The model under review builds one solid part; all positions refer to its coordinate system, in mm. A direction names the side the tool comes from. Give positions to 0.01 mm unless a question says otherwise; leave off trailing zeros. Loops run counter-clockwise (first coordinate to the right, second up) from the corner with the lowest first, then second, coordinate; pieces in that order, holes last. Notation, with made-up numbers: M 22.5,28 L 28.5,28 A16 ccw 28.5,47 Z; hole C 28,-17 d10. An arc over 180 degrees is marked long. Write item = value, one per line. Start each with the question number.
1. We need section B-B on x = 7.5. Give the boundary of the cut face in (y, z).
2. Draft analysis for pull direction X (two halves, no side actions). For faces 6 (the face through (0, 1.5, 0)), 7 (the face through (0.1, 7.6, 0)), 8 (the face through (8.7, 2.34, -0.05)), 9 (the face through (-6.3, 2.34, -0.05)), state which applies: pulls with the +X half, pulls with the -X half, needs draft (parallel to the pull), parting line crosses it, or undercut.
3. Wall thickness on line 1 along Z through (x, y) = (-7.5, 2.45); line 2 along X through (y, z) = (4.5, -0.75); line 3 along X through (y, z) = (1, -0.75): over which ranges is each line inside the solid? List them lowest first. Write a range as from..to.
4. We need section C-C on z = -2.25. Give the boundary of the cut face in (x, y).
5. We need section A-A on x = -9. Give the boundary of the cut face in (y, z), then the cut area to 3 significant figures.
6. We need section D-D on y = 4.25. Give the boundary of the cut face in (x, z), then the cut area to 3 significant figures.
7. For faces 1 (the face through (6, 3.1, 0)), 2 (the face through (-2, 1, -3)), 3 (the face through (0, 6.1, 0)), 4 (the face through (0, 0, 0)), 5 (the face through (-9, 3.1, 0)), list the 3-axis set-ups (+Z, -Z, +X, -X, +Y, -Y) from which the entire face can be reached by the end or side of a thin tool; tool diameter is ignored.
8. For pin 1 (1.8 mm diameter, centred on x = 7, z = 0, fed in from +Y); pin 2 (1 mm diameter, centred on y = 5, z = -0.5, fed in from +X), all flat-tipped, find the tip position at first contact; note any pin that passes through.
from build123d import *

# Parameters (mm, degrees)
BOSS_EXTRUDE1_DEPTH  = 3
M2_CLEARANCE_HOLE1_D = 2.4
FILLET1_R            = 2


with BuildPart() as part:
    # Sketch1 → Boss-Extrude1 (new, symmetric)
    with BuildSketch(Plane.XY):
        with BuildLine():
            ThreePointArc((4.5, 3.1), (3.439339828, 3.539339828), (3, 4.6))
            ThreePointArc((3, 4.6), (2.121320344, 6.721320344), (0, 7.6))
            ThreePointArc((0, 7.6), (-2.121320344, 6.721320344), (-3, 4.6))
            ThreePointArc((-3, 4.6), (-3.439339828, 3.539339828), (-4.5, 3.1))
            Line((-4.5, 3.1), (-10.5, 3.1))
            ThreePointArc((-10.5, 3.1), (-12.05, 1.55), (-10.5, 0))
            Line((-10.5, 0), (10.7, 0))
            Line((10.7, 0), (10.7, 1.5))
            Line((10.7, 1.5), (-10.5, 1.5))
            ThreePointArc((-10.5, 1.5), (-10.55, 1.55), (-10.5, 1.6))
            Line((-10.5, 1.6), (-4.5, 1.6))
            ThreePointArc((-4.5, 1.6), (-2.378679656, 2.478679656), (-1.5, 4.6))
            ThreePointArc((-1.5, 4.6), (-1.060660172, 5.660660172), (0, 6.1))
            ThreePointArc((0, 6.1), (1.060660172, 5.660660172), (1.5, 4.6))
            ThreePointArc((1.5, 4.6), (2.378679656, 2.478679656), (4.5, 1.6))
            Line((4.5, 1.6), (10.7, 1.6))
            Line((10.7, 1.6), (10.7, 3.1))
            Line((10.7, 3.1), (4.5, 3.1))
        make_face()
    extrude(amount=BOSS_EXTRUDE1_DEPTH, both=True)

    # M2 Clearance Hole1 (through all)
    with Locations(Plane(origin=(0, 3.1, 0), x_dir=(1, 0, 0), z_dir=(0, 1, 0))):
        with Locations((-7.5, 0), (7.5, 0)):
            Hole(M2_CLEARANCE_HOLE1_D / 2)

    # Fillet1
    fillet1_edges = [part.edges().sort_by_distance(p)[0] for p in [
        (10.7, 2.35, -3),
        (10.7, 0.75, -3),
        (10.7, 0.75, 3),
        (10.7, 2.35, 3),
    ]]
    fillet(fillet1_edges, radius=FILLET1_R)


solid = part.part
Final values:
q1.outline = M 0,-3 L 1.5,-3 L 1.5,-1.2 L 0,-1.2 Z; M 0,1.2 L 1.5,1.2 L 1.5,3 L 0,3 Z; M 1.6,-3 L 3.1,-3 L 3.1,-1.2 L 1.6,-1.2 Z; M 1.6,1.2 L 3.1,1.2 L 3.1,3 L 1.6,3 Z
q2.face_6 = needs draft
q2.face_7 = parting line crosses it
q2.face_8 = undercut
q2.face_9 = undercut
q3.line_1 = -3..-1.2, 1.2..3
q3.line_2 = -3..-1.5, 1.5..3
q3.line_3 = -11.95..-8.44, -6.56..6.56, 8.44..10.7
q4.outline = M -10.5,0 L 10.26,0 L 10.26,1.5 L -10.5,1.5 A0.05 cw -10.5,1.6 L -4.5,1.6 A3 ccw -1.5,4.6 A1.5 cw 1.5,4.6 A3 ccw 4.5,1.6 L 10.26,1.6 L 10.26,3.1 L 4.5,3.1 A1.5 cw 3,4.6 A3 ccw -3,4.6 A1.5 cw -4.5,3.1 L -10.5,3.1 A1.55 ccw Z
q5.outline = M 0,-3 L 1.5,-3 L 1.5,3 L 0,3 Z; M 1.6,-3 L 3.1,-3 L 3.1,3 L 1.6,3 Z
q5.area = 18.0 mm²
q6.outline = M -3.04,-3 L -1.52,-3 L -1.52,3 L -3.04,3 Z; M 1.52,-3 L 3.04,-3 L 3.04,3 L 1.52,3 Z
q6.area = 18.3 mm²
q7.face_1 = +Z, -Z, +X, +Y
q7.face_2 = -Z, +X, -X, +Y, -Y
q7.face_3 = +Z, -Z
q7.face_4 = +Z, -Z, +X, -X, -Y
q7.face_5 = +Z, -Z, -X, +Y
q8.pin_1 = 3.1
q8.pin_2 = 3
